```python
from build123d import *

# Parameters (mm, degrees)
EXTRUDE_1_OUTLINE_R   = 76
EXTRUDE_1_OUTLINE_R_2 = 0.65
EXTRUDE_1_OUTLINE_R_3 = 68
EXTRUDE_1_DEPTH       = 3
SKETCH_2_W            = 11
SKETCH_2_H            = 4
EXTRUDE_2_DEPTH       = 2
SKETCH_3_R            = 0.6
EXTRUDE_3_DEPTH       = 3


# Read off the part's stored shape, not the designer's step: 凸台-拉伸1
with BuildPart() as part:
    # 凸台-拉伸1 outline → 凸台-拉伸1 (new body)
    with BuildSketch(Plane.XY):
        Circle(EXTRUDE_1_OUTLINE_R)
        with Locations((-53, -53)):
            Circle(EXTRUDE_1_OUTLINE_R_2, mode=Mode.SUBTRACT)
        with Locations((53, -53)):
            Circle(EXTRUDE_1_OUTLINE_R_2, mode=Mode.SUBTRACT)
        with Locations((-53, 53)):
            Circle(EXTRUDE_1_OUTLINE_R_2, mode=Mode.SUBTRACT)
        Circle(EXTRUDE_1_OUTLINE_R_3, mode=Mode.SUBTRACT)
        with Locations((53, 53)):
            Circle(EXTRUDE_1_OUTLINE_R_2, mode=Mode.SUBTRACT)
    extrude(amount=EXTRUDE_1_DEPTH)

    # 草图2 → 凸台-拉伸2 (add)
    with BuildSketch(Plane.XY.offset(3)):
        with Locations((0, 72)):
            Rectangle(SKETCH_2_W, SKETCH_2_H)
    extrude(amount=EXTRUDE_2_DEPTH)

    # 草图3 → 凸台-拉伸3 (add)
    with BuildSketch(Plane(origin=(0, 74, 0), x_dir=(1, 0, 0), z_dir=(0, 1, 0))):
        with Locations(Location((-1.5, -4, 0), (0, 0, 90))):
            Circle(SKETCH_3_R)
        with Locations(Location((1.5, -4, 0), (0, 0, 90))):
            Circle(SKETCH_3_R)
        with Locations(Location((-4, -4, 0), (0, 0, 90))):
            Circle(SKETCH_3_R)
        with Locations(Location((4, -4, 0), (0, 0, 90))):
            Circle(SKETCH_3_R)
    extrude(amount=EXTRUDE_3_DEPTH)


solid = part.part
```
The listing builds one solid part. Answer for the finished solid, in the listing's coordinates (mm). Give positions to 0.01 mm unless a question says otherwise; leave off trailing zeros. Order: outer loops, then holes, each group sorted by start corner. A loop starts at its lowest first (then second) coordinate and runs counter-clockwise, first axis right, second up. Notation, with made-up numbers: (-8, 38) -> (28, 38) arc R37 ccw to (28, 77) -> close; hole circle Ø4 at (80, 45.25). An arc over 180 degrees is marked (long way). Answer as a JSON object with one key per item and string values. Group by question number.
Item 1: The part is cut by section C-C on z = 0.8. Write down the section's boundary in (x, y).
Item 2: The part is cut by section B-B on x = -46. Write down the section's boundary in (y, z).
Item 3: Consider L1, parallel to X at y = -1.5, z = 0.4; L2, parallel to Y at x = 53, z = 1.55. Determine where each line is inside the solid, lowest interval first. Write a range as from..to.
Item 4: The part is cut by section A-A on y = -30. Write down the section's boundary in (x, z), and give its area (3 significant figures).
Item 5: Determine the mould class of faces 1 (the cylindrical face through (36.556, 57.338, 1.479)), 2 (the flat face through (0, 72, 5)), 3 (the cylindrical face through (35.069, -67.425, 1.479)) for opening direction Y: pulls with the +Y half, pulls with the -Y half, needs draft (parallel to the pull), parting line crosses it, or undercut.
Item 6: Flat-ended cylindrical pins translate along their axes: pin 1 (0.8 mm diameter, centred on x = 53, y = -53, fed in from +Z); pin 2 (3 mm diameter, centred on x = -8, z = 2.5, fed in from +Y); pin 3 (1.5 mm diameter, centred on y = 7, z = 2, fed in from -X); pin 4 (1 mm diameter, centred on y = 72, z = 4, fed in from -X). Find the tip coordinate at first contact, or state that the pin passes through.
Result set:
{
 "1": {"outline": "circle Ø152 at (0, 0); hole circle Ø136 at (0, 0); hole circle Ø1.3 at (-53, -53); hole circle Ø1.3 at (-53, 53); hole circle Ø1.3 at (53, -53); hole circle Ø1.3 at (53, 53)"},
 "2": {"outline": "(-60.5, 0) -> (-50.08, 0) -> (-50.08, 3) -> (-60.5, 3) -> close; (50.08, 0) -> (60.5, 0) -> (60.5, 3) -> (50.08, 3) -> close"},
 "3": {"L1": "-75.99..-67.98, 67.98..75.99", "L2": "-54.47..-53.65, -52.35..-42.6, 42.6..52.35, 53.65..54.47"},
 "4": {"outline": "(-69.83, 0) -> (-61.02, 0) -> (-61.02, 3) -> (-69.83, 3) -> close; (61.02, 0) -> (69.83, 0) -> (69.83, 3) -> (61.02, 3) -> close", "area": "52.8 mm²"},
 "5": {"face 1": "undercut", "face 2": "needs draft", "face 3": "parting line crosses it"},
 "6": {"pin 1": "through", "pin 2": "y = 75.72", "pin 3": "x = -75.74", "pin 4": "x = -5.5"}
}
